Geometry check sheet. Reference: the model listing, model coordinates, mm. A direction names the side the tool comes from. Give positions to 0.01 mm unless a question says otherwise; leave off trailing zeros. Loops run counter-clockwise (first coordinate to the right, second up) from the corner with the lowest first, then second, coordinate; pieces in that order, holes last. Notation, with made-up numbers: (13.5, 35.5) - (65.5, 35.5) arc R20 cw to (65.5, 73.5) - close; hole circle Ø7 at (-22, 33). An arc over 180 degrees is marked (long way). Use a Markdown table: item, result. Add a question column.
1. Material ranges on L1, parallel to Y at x = 8.5, z = 0.25; L2, parallel to Y at x = 23.5, z = -0.1; L3, parallel to Y at x = 47, z = 0.7, recorded low to high.
2. Cross-section at D-D on y = -19.5. Enter the section's corners in (x, z), and give its area (3 significant figures).
3. Cross-section at B-B on y = 17.78. Enter the section's corners in (x, z).
4. Cross-section at A-A on z = 0. Enter the section's corners in (x, y).
5. Set-up check for faces 1 (the cylindrical face through (0, 17.9, 0)), 2 (the flat face through (22, 22.098, 0)), 3 (the flat face through (48, 5.08, 0)): record each of +Z, -Z, +X, -X, +Y, -Y from which the full face is reachable in a straight line by a thin tool's end or side.
6. Cross-section at C-C on x = 11. Enter the section's corners in (y, z), and give its area (3 significant figures).
7. Depth check by flat-ended pin: P1, Ø1, axis at x = 19.5, z = 0, coming from the -Y side; P2, Ø0.6, axis at x = 50, z = -0.5, coming from the -Y side; P3, Ø2.5, axis at x = 6.731, y = 17.78, coming from the -Z side. Enter the tip coordinate at first touch or a pass-through.
from build123d import *

# Parameters (mm, degrees)
F0_R     = 2.159
F1_DEPTH = 1.016


with BuildPart() as f1:
    # F0 (on Top) → F1 (new body, symmetric)
    with BuildSketch(Plane.XY):
        with BuildLine():
            Line((13.208, 22.098), (4.318, 22.098))
            ThreePointArc((4.318, 22.098), (0, 17.78), (4.318, 13.462))
            Line((4.318, 13.462), (24.892, 13.462))
            Line((24.892, 13.462), (41.098512, 10.321209))
            ThreePointArc((41.098512, 10.321209), (44.050946, 8.566377), (45.212, 5.334))
            Line((45.212, 5.334), (45.212, 5.08))
            Line((45.212, 5.08), (51.562, 5.08))
            ThreePointArc((51.562, 5.08), (84.679548, -4.563853), (107.442, -30.48))
            ThreePointArc((107.442, -30.48), (92.910204, 12.290854), (51.562, 30.48))
            Line((51.562, 30.48), (45.212, 30.48))
            Line((45.212, 30.48), (45.212, 30.226))
            ThreePointArc((45.212, 30.226), (44.050946, 26.993623), (41.098512, 25.238791))
            Line((41.098512, 25.238791), (24.892, 22.098))
            Line((24.892, 22.098), (19.05, 22.098))
            ThreePointArc((19.05, 22.098), (16.129, 19.177), (13.208, 22.098))
        make_face()
        with Locations((6.731, 17.78)):
            Circle(F0_R, mode=Mode.SUBTRACT)
    extrude(amount=F1_DEPTH, both=True)


solid = f1.part
Values found:
| question | item | result |
|---|---|---|
| 1 | L1 | y = 13.46 to 16.54, 19.02 to 22.1 |
| 1 | L2 | y = 13.46 to 22.1 |
| 1 | L3 | y = 5.08 to 30.48 |
| 2 | outline | (100.84, -1.02) - (107.32, -1.02) - (107.32, 1.02) - (100.84, 1.02) - close |
| 2 | area | 13.2 mm2 |
| 3 | outline | (0, -1.02) - (4.57, -1.02) - (4.57, 1.02) - (0, 1.02) - close; (8.89, -1.02) - (87.11, -1.02) - (87.11, 1.02) - (8.89, 1.02) - close |
| 4 | outline | (4.32, 13.46) - (24.89, 13.46) - (41.1, 10.32) arc R5.08 cw to (45.21, 5.33) - (45.21, 5.08) - (51.56, 5.08) arc R61.69 cw to (107.44, -30.48) arc R56.09 ccw to (51.56, 30.48) - (45.21, 30.48) - (45.21, 30.23) arc R5.08 cw to (41.1, 25.24) - (24.89, 22.1) - (19.05, 22.1) arc R2.92 cw to (13.21, 22.1) - (4.32, 22.1) arc R4.32 ccw to start; hole circle Ø4.32 at (6.73, 17.78) |
| 5 | face 1 | +Z, -Z, -X |
| 5 | face 2 | +Z, -Z, -X, +Y |
| 5 | face 3 | +Z, -Z, -X, -Y |
| 6 | outline | (13.46, -1.02) - (22.1, -1.02) - (22.1, 1.02) - (13.46, 1.02) - close |
| 6 | area | 17.5 mm2 |
| 7 | P1 | stops at y = 13.46 |
| 7 | P2 | stops at y = 5.08 |
| 7 | P3 | passes through |
